Part model, mm, in its own coordinate system. A direction names the side the tool comes from. Give positions to 0.01 mm unless a question says otherwise; leave off trailing zeros. Write each loop counter-clockwise with the first axis right and the second up, starting at its lowest first coordinate (ties: lowest second). Pieces come first, ordered by that corner, then holes. Notation, with made-up numbers: M 47.5,-11.5 L 99.5,-11.5 A24 cw 99.5,21.5 Z; hole C 18,2.25 d2. An arc over 180 degrees is marked long. Answer as CSV lines item,"result". Start each with the question number.
1) Mould opens along X. For faces 3 (the flat face through (1.5, 5, 9)), 4 (the flat face through (-3, 6, -3)), 5 (the cylindrical face through (14.985, 2.958, -0.66)) say: pulls with the +X half, pulls with the -X half, needs draft (parallel to the pull), parting line crosses it, or undercut.
2) Wall check: line 1 along X through (y, z) = (1.45, 0); line 2 along Z through (x, y) = (1.75, 2). Give the ranges that are in metal, low to high. Write a range as from..to.
3) Slice it at C-C, the plane y = 0.9. Give the cut face in (x, z), plus the area to 3 significant figures.
4) Slice it at A-A, the plane x = 0. Give the cut face in (y, z).
5) Tool access for faces 1 (the flat face through (-1.5, 5, 9)), 2 (the cylindrical face through (2.15, 3.042, -3.373)): list every direction of +Z, -Z, +X, -X, +Y, -Y with a clear straight run to the whole face (end or side of a thin tool).
6) Pin check, flat tips, straight feed: pin 1 Ø1 at (y, z) = (3, 6) entering from -X; pin 2 Ø3 at (x, y) = (-9, 5) entering from -Z; pin 3 Ø1.5 at (x, z) = (0, 10.5) entering from +Y. Stop position of each tip, or through.
7) Slice it at D-D, the plane z = 7.5. Give the cut face in (x, y), plus the area to 3 significant figures.
8) Slice it at B-B, the plane z = 0. Give the cut face in (x, y).
Autodesk Inventor part; units mm, degrees
ref_plane "YZ Plane" through (0, 0, 0) normal (1, 0, 0) x (0, 1, 0)
ref_plane "XZ Plane" through (0, 0, 0) normal (0, 1, 0) x (-1, 0, 0)
ref_plane "XY Plane" through (0, 0, 0) normal (0, 0, 1) x (1, 0, 0)
sketch "スケッチ1" plane through (0, 0, 0) normal (0, 1, 0) x (-1, 0, 0)
  circle A0 centre (0, 0) radius 15
  dimension "d0" = 30
extrude "押し出し1" add sketch "スケッチ1" along normal blind 6
sketch "スケッチ2" plane through (0, 6, 0) normal (0, 1, 0) x (1, 0, 0)
  circle A0 centre (0, 0) radius 3
  dimension "d3" = 6
extrude "押し出し2" cut sketch "スケッチ2" against normal blind 6
sketch "スケッチ3" plane through (0, 6, 0) normal (0, 1, 0) x (1, 0, 0)
  line L0 (-1.5, 0) -> (1.5, 0)
  line L1 (1.5, 0) -> (1.5, -17.8431)
  line L2 (1.5, -17.8431) -> (-1.5, -17.8431)
  line L3 (-1.5, -17.8431) -> (-1.5, 0)
  point P0 (0, 0)
  dimension "d6" = 3
  dimension "d7" = 1.5
extrude "押し出し3" cut sketch "スケッチ3" against normal blind 3
sketch "スケッチ4" plane through (0, 6, 0) normal (0, 1, 0) x (1, 0, 0)
  circle A0 centre (0, 0) radius 4
  dimension "d10" = 8
extrude "押し出し4" cut sketch "スケッチ4" against normal blind 6
properties part number "NHK_t0_1"
Found:
1,face 3,"undercut"
1,face 4,"needs draft"
1,face 5,"parting line crosses it"
2,line 1,"-15..-4, 4..15"
2,line 2,"-14.9..-3.6, 3.6..14.9"
3,outline,"C 0,0 d30; hole C 0,0 d8"
3,area,"657 mm²"
4,outline,"M 0,-15 L 6,-15 L 6,-4 L 0,-4 Z; M 0,4 L 3,4 L 3,15 L 0,15 Z"
5,face 1,"+Z, +Y"
5,face 2,"+Y, -Y"
6,pin 1,"x = -13.96"
6,pin 2,"z = -12.99"
6,pin 3,"y = 3"
7,outline,"M -12.99,0 L 12.99,0 L 12.99,6 L 1.5,6 L 1.5,3 L -1.5,3 L -1.5,6 L -12.99,6 Z"
7,area,"147 mm²"
8,outline,"M -15,0 L -4,0 L -4,6 L -15,6 Z; M 4,0 L 15,0 L 15,6 L 4,6 Z"
